from build123d import *

# Parameters (mm, degrees)
F1_DEPTH     = 8
F2_W         = 2.5
F2_H         = 12.5
F3_DEPTH     = 4
F4_W         = 7.3
F4_H         = 12.5
F5_DEPTH     = 2
F7_DEPTH     = 2
F9_DEPTH     = 2
F10_T1_DEPTH = 8
F11_R        = 2.15
F12_DEPTH    = 2.5


# Not quite as in the source:
# - a fillet or chamfer that OpenCascade refuses, or shapes differently, is made with other operations: its cross-section is extruded or revolved along the edge and cut away or added


with BuildPart() as f1:
    # F0 (on Top) → F1 (new body)
    with BuildSketch(Plane.XY):
        Polygon((87.45, 92), (-87.45, 92), (-87.45, 86), (-46.45, 86), (-46.45, 73.5), (-43.95, 73.5), (-43.95, 86), (-41.65, 86), (-41.65, 73.5), (-39.15, 73.5), (-39.15, 86), (-35.15, 86), (-35.15, 0), (-35.15, -86), (-39.15, -86), (-39.15, -73.5), (-41.65, -73.5), (-41.65, -86), (-43.95, -86), (-43.95, -73.5), (-46.45, -73.5), (-46.45, -86), (-87.45, -86), (-87.45, -92), (87.45, -92), (87.45, 0), align=None)
        Polygon((-29.15, -86), (-29.15, 0), (-29.15, 86), (11.85, 86), (11.85, 73.5), (14.35, 73.5), (14.35, 86), (16.65, 86), (16.65, 73.5), (19.15, 73.5), (19.15, 86), (23.15, 86), (23.15, 0), (23.15, -86), (19.15, -86), (19.15, -73.5), (16.65, -73.5), (16.65, -86), (14.35, -86), (14.35, -73.5), (11.85, -73.5), (11.85, -86), align=None, mode=Mode.SUBTRACT)
        Polygon((29.15, -86), (29.15, 0), (29.15, 86), (70.15, 86), (70.15, 73.5), (72.65, 73.5), (72.65, 86), (74.95, 86), (74.95, 73.5), (77.45, 73.5), (77.45, 86), (81.45, 86), (81.45, 0), (81.45, -86), (77.45, -86), (77.45, -73.5), (74.95, -73.5), (74.95, -86), (72.65, -86), (72.65, -73.5), (70.15, -73.5), (70.15, -86), align=None, mode=Mode.SUBTRACT)
    extrude(amount=F1_DEPTH)

    # F2 (on face) → F3 (join)
    with BuildSketch(Plane.XY.offset(8)):
        with Locations((-40.4, 79.75)):
            Rectangle(F2_W, F2_H)
        with Locations((-45.2, 79.75)):
            Rectangle(F2_W, F2_H)
        with Locations((13.1, 79.75)):
            Rectangle(F2_W, F2_H)
        with Locations((17.9, 79.75)):
            Rectangle(F2_W, F2_H)
        with Locations((76.2, 79.75)):
            Rectangle(F2_W, F2_H)
        with Locations((71.4, 79.75)):
            Rectangle(F2_W, F2_H)
        with Locations((76.2, -79.75)):
            Rectangle(F2_W, F2_H)
        with Locations((71.4, -79.75)):
            Rectangle(F2_W, F2_H)
        with Locations((-40.4, -79.75)):
            Rectangle(F2_W, F2_H)
        with Locations((-45.2, -79.75)):
            Rectangle(F2_W, F2_H)
        with Locations((17.9, -79.75)):
            Rectangle(F2_W, F2_H)
        with Locations((13.1, -79.75)):
            Rectangle(F2_W, F2_H)
    extrude(amount=F3_DEPTH)

    # F4 (on face) → F5 (join)
    with BuildSketch(Plane(origin=(0, 0, 0), x_dir=(1, 0, 0), z_dir=(0, 0, -1))):
        with Locations((-42.8, 79.75)):
            Rectangle(F4_W, F4_H)
        with Locations((15.5, 79.75)):
            Rectangle(F4_W, F4_H)
        with Locations((73.8, 79.75)):
            Rectangle(F4_W, F4_H)
        with Locations((15.5, -79.75)):
            Rectangle(F4_W, F4_H)
        with Locations((-42.8, -79.75)):
            Rectangle(F4_W, F4_H)
        with Locations((73.8, -79.75)):
            Rectangle(F4_W, F4_H)
    extrude(amount=-F5_DEPTH)

    # F6 (on face) → F7 (cut)
    with BuildSketch(Plane.XY.offset(8)):
        Polygon((85.45, 90), (-85.45, 90), (-85.45, 88), (-33.15, 88), (-33.15, 0), (-33.15, -88), (-85.45, -88), (-85.45, -90), (85.45, -90), (85.45, 0), align=None)
        Polygon((25.15, 88), (25.15, 0), (25.15, -88), (-31.15, -88), (-31.15, 0), (-31.15, 88), align=None, mode=Mode.SUBTRACT)
        Polygon((27.15, 88), (83.45, 88), (83.45, 0), (83.45, -88), (27.15, -88), (27.15, 0), align=None, mode=Mode.SUBTRACT)
    extrude(amount=-F7_DEPTH, mode=Mode.SUBTRACT)

    # F8 (on face) → F9 (cut)
    with BuildSketch(Plane(origin=(0, 0, 0), x_dir=(1, 0, 0), z_dir=(0, 0, -1))):
        Polygon((85.45, 90), (-85.45, 90), (-85.45, 88), (-33.15, 88), (-33.15, 0), (-33.15, -88), (-85.45, -88), (-85.45, -90), (85.45, -90), (85.45, 0), align=None)
        Polygon((25.15, 88), (25.15, 0), (25.15, -88), (-31.15, -88), (-31.15, 0), (-31.15, 88), align=None, mode=Mode.SUBTRACT)
        Polygon((27.15, 88), (83.45, 88), (83.45, 0), (83.45, -88), (27.15, -88), (27.15, 0), align=None, mode=Mode.SUBTRACT)
    extrude(amount=-F9_DEPTH, mode=Mode.SUBTRACT)

    # F10: chamfer of 5 on 12 edges, made by hand

    # F10_s2 → F10_t1 (join)
    with BuildSketch(Plane.XY):
        Polygon((-39.15, 81), (-34.15, 86), (-39.15, 86), align=None)
        Polygon((-51.45, 86), (-46.45, 81), (-46.45, 86), align=None)
        Polygon((11.85, 81), (6.85, 86), (11.85, 86), align=None)
        Polygon((24.15, 86), (19.15, 81), (19.15, 86), align=None)
        Polygon((77.45, 81), (82.45, 86), (77.45, 86), align=None)
        Polygon((65.15, 86), (70.15, 81), (70.15, 86), align=None)
        Polygon((77.45, -81), (82.45, -86), (77.45, -86), align=None)
        Polygon((65.15, -86), (70.15, -81), (70.15, -86), align=None)
        Polygon((11.85, -81), (6.85, -86), (11.85, -86), align=None)
        Polygon((-51.45, -86), (-46.45, -81), (-46.45, -86), align=None)
        Polygon((-39.15, -81), (-34.15, -86), (-39.15, -86), align=None)
        Polygon((24.15, -86), (19.15, -81), (19.15, -86), align=None)
    extrude(amount=F10_T1_DEPTH)

    # F11 (on face) → F12 (join)
    with BuildSketch(Plane(origin=(0, 0, 0), x_dir=(1, 0, 0), z_dir=(0, 0, -1))):
        Polygon((29.15, -52.7659812842), (29.15, -86), (62.3840187158, -86), align=None)
        with Locations((37.4585046789, -77.6914953211)):
            Circle(F11_R, mode=Mode.SUBTRACT)
        Polygon((29.15, 86), (29.15, 52.7659812842), (62.3840187158, 86), align=None)
        with Locations((37.4585046789, 77.6914953211)):
            Circle(F11_R, mode=Mode.SUBTRACT)
        Polygon((-29.15, -52.7659812842), (-29.15, -86), (4.0840187158, -86), align=None)
        with Locations((-20.8414953211, -77.6914953211)):
            Circle(F11_R, mode=Mode.SUBTRACT)
        Polygon((-29.15, 86), (-29.15, 52.7659812842), (4.0840187158, 86), align=None)
        with Locations((-20.8414953211, 77.6914953211)):
            Circle(F11_R, mode=Mode.SUBTRACT)
    extrude(amount=-F12_DEPTH)


solid = f1.part
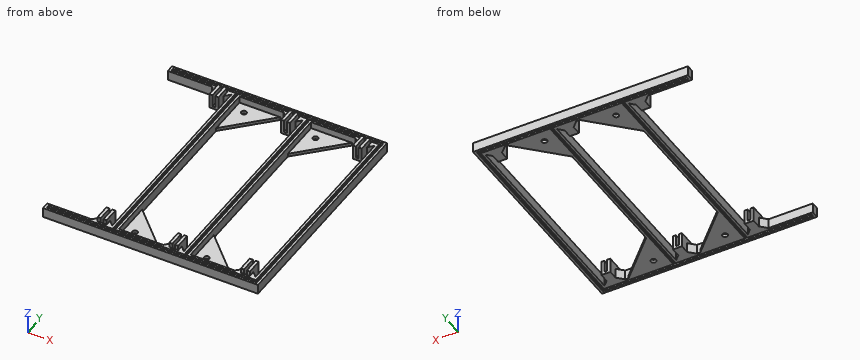
Input: part model. Units: mm. Frame: model coordinates. Round coordinates to 2 decimals unless told otherwise and drop trailing zeros. Order: outer loops, then holes, each group sorted by start corner. A loop starts at its lowest first (then second) coordinate and runs counter-clockwise, first axis right, second up.
1. Cut plane C-C, the plane x = 48.5. Output: boundary loops of the cut face in (y, z), then the cut area to 3 significant figures.
The answers:
outline: (-92, 0) - (-90, 0) - (-90, 2) - (-88, 2) - (-88, 0) - (-72.12, 0) - (-72.12, 2.5) - (-86, 2.5) - (-86, 8) - (-88, 8) - (-88, 6) - (-90, 6) - (-90, 8) - (-92, 8) - close; (72.12, 0) - (88, 0) - (88, 2) - (90, 2) - (90, 0) - (92, 0) - (92, 8) - (90, 8) - (90, 6) - (88, 6) - (88, 8) - (86, 8) - (86, 2.5) - (72.12, 2.5) - close
area: 149 mm2
2. Cut plane A-A, the plane x = -75. Output: boundary loops of the cut face in (y, z).
The answers:
outline: (-92, 0) - (-90, 0) - (-90, 2) - (-88, 2) - (-88, 0) - (-86, 0) - (-86, 8) - (-88, 8) - (-88, 6) - (-90, 6) - (-90, 8) - (-92, 8) - close; (86, 0) - (88, 0) - (88, 2) - (90, 2) - (90, 0) - (92, 0) - (92, 8) - (90, 8) - (90, 6) - (88, 6) - (88, 8) - (86, 8) - close
3. Cut plane B-B, the plane y = -47.5. State how many separate pieces and enclosed holes the cut face has, then the cut area to 3 significant figures.
The answers:
separate pieces: 3
enclosed holes: 0
area: 120 mm2
4. Material intervals for line 1 (X direction, y = 28, z = 6.75); line 2 (Y direction, x = 15.5, z = 7); line 3 (X direction, y = -39, z = 2.25), sorted ascending.
The answers:
line 1: x = -35.15 to -33.15, -31.15 to -29.15, 23.15 to 25.15, 27.15 to 29.15, 81.45 to 83.45, 85.45 to 87.45
line 2: y = -92 to -90, -88 to -86, 86 to 88, 90 to 92
line 3: x = -35.15 to -29.15, 23.15 to 29.15, 81.45 to 87.45
5. Cut plane D-D, the plane x = -1.5. Output: boundary loops of the cut face in (y, z).
The answers:
outline: (-92, 0) - (-90, 0) - (-90, 2) - (-88, 2) - (-88, 0) - (-80.42, 0) - (-80.42, 2.5) - (-86, 2.5) - (-86, 8) - (-88, 8) - (-88, 6) - (-90, 6) - (-90, 8) - (-92, 8) - close; (80.42, 0) - (88, 0) - (88, 2) - (90, 2) - (90, 0) - (92, 0) - (92, 8) - (90, 8) - (90, 6) - (88, 6) - (88, 8) - (86, 8) - (86, 2.5) - (80.42, 2.5) - close
6. Pin query (flat end, axial travel): P1, Ø5, axis at x = 37.46, y = 77.69, coming from the +Z side; P2, Ø6, axis at x = -23.5, y = -45.5, coming from the -Z side; P3, Ø6, axis at x = 63, z = 10, coming from the -Y side; P4, Ø2, axis at x = -45, z = 10, coming from the +Y side. Return the tip coordinate at first contact, or that it passes through.
The answers:
P1: stops at z = 2.5
P2: passes through
P3: stops at y = -92
P4: stops at y = 86
